Autodesk Inventor part; units mm, degrees
ref_plane "YZ Plane" through (0, 0, 0) normal (1, 0, 0) x (0, 1, 0)
ref_plane "XZ Plane" through (0, 0, 0) normal (0, 1, 0) x (-1, 0, 0)
ref_plane "XY Plane" through (0, 0, 0) normal (0, 0, 1) x (1, 0, 0)
sketch "Sketch1" plane through (0, 0, 0) normal (0, 0, 1) x (1, 0, 0)
  line L0 (-127, 635) -> (127, 635)
  line L1 (127, 635) -> (127, -635)
  line L2 (127, -635) -> (-127, -635)
  line L3 (-127, -635) -> (-127, 635)
  line L4 (-127, 635) -> (127, -635) construction
  line L5 (127, 635) -> (-127, -635) construction
  point P0 (0, 0)
  dimension "d0" = 254
  dimension "d1" = 1270
extrude "Extrusion1" add sketch "Sketch1" along normal blind 25.4
sketch "Sketch2" plane through (0, 0, 25.4) normal (0, 0, 1) x (1, 0, 0)
  line L0 (127, 635) -> (-127, 635)
  line L1 (-63.5, -381) -> (63.5, -381)
  line L2 (63.5, -381) -> (63.5, -508)
  line L3 (63.5, -508) -> (-63.5, -508)
  line L4 (-63.5, -508) -> (-63.5, -381)
  line L5 (-63.5, -381) -> (63.5, -508) construction
  line L6 (63.5, -381) -> (-63.5, -508) construction
  line L7 (0, 635) -> (0, 508)
  point P0 (0, 0)
  dimension "d5" = 127
  dimension "d6" = 127
  dimension "d7" = 127
hole "Hole1" at (0, 508, 25.4) direction (0, 0, -1) diameter 6.35 end through all
extrude "Extrusion2" add sketch "Sketch2" along normal blind 254
sketch "Sketch3" plane through (-63.5, -381, 25.4) normal (0, 1, 0) x (1, 0, 0)
  line L0 (127, -254) -> (0, -254)
  line L1 (127, 0) -> (127, -254)
  line L2 (63.5, -254) -> (63.5, -50.8)
  point P0 (63.5, 25.4)
  dimension "d17" = 203.2
hole "Hole2" at (0, -381, 76.2) direction (0, -1, 0) diameter 6.35 end through all
sketch "Sketch4" plane through (-63.5, -381, 25.4) normal (0, 1, 0) x (1, 0, 0)
  circle A0 centre (63.5, -50.8) radius 3.175
  line L0 (0, 0) -> (127, 0)
  line L1 (0, 0) -> (0, -254)
  line L2 (127, -254) -> (0, -254)
  line L3 (127, 0) -> (127, -254)
  point P0 (63.5, 25.4)
  point P1 (63.5, -53.975)
properties part number "base"
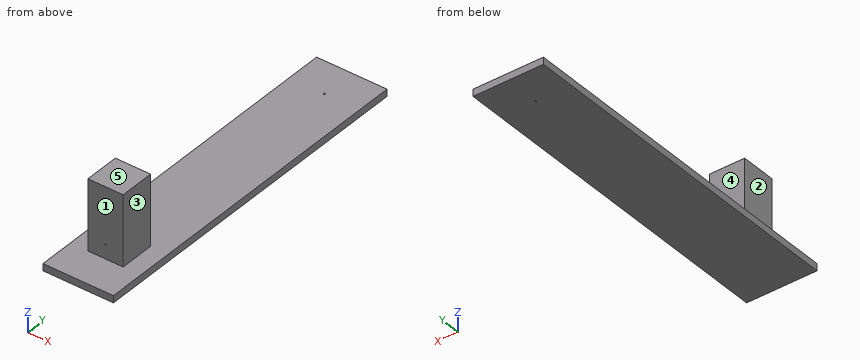
Input: part model. Units: mm. Frame: model coordinates. Face numbers are marked on the shaded views. A direction names the side the tool comes from. Coordinates: 2 decimals unless noted, no trailing zeros. Order: outer loops, then holes, each group sorted by start corner. A loop starts at its lowest first (then second) coordinate and runs counter-clockwise, first axis right, second up. Notation, with made-up numbers: M 36.5,81 L 58.5,81 A10 ccw 58.5,94 Z; hole C -29.75,15 d4. An arc over 180 degrees is marked long. Write item = value, one per line. Start each with the question number.
(1) Section D-D on y = -347.5. Output: boundary loops of the cut face in (x, z).
(2) Section A-A on y = -491.5. Output: boundary loops of the cut face in (x, z) (3 decimals), and give its area (3 significant figures).
(3) Line query: line 1 along Y through (x, z) = (0, 20) (3 decimals); line 2 along X through (y, z) = (508, 8.75) (3 decimals); line 3 along Z through (x, y) = (42, 519.5). Output: solid intervals per line, ascending. Write a range as [from, to].
(4) First-contact query: P1, Ø3, axis at x = 0.5, y = -244, coming from the +Z side. Flat tip, straight axial feed; report the tip coordinate or a pass-through.
(5) Section C-C on z = 216.5. Output: boundary loops of the cut face in (x, y).
(6) Reachability of the marked faces 1, 2, 3, 4 and 5 from +Z, -Z, +X, -X, +Y, -Y: full face, straight path, thin tool, end or side. Return the list, or none.
(7) Section B-B on x = -31. Output: boundary loops of the cut face in (y, z), and give its area (3 significant figures).
Result set:
q1.outline = M -127,0 L 127,0 L 127,25.4 L -127,25.4 Z
q2.outline = M -127,0 L 127,0 L 127,25.4 L 63.5,25.4 L 63.5,279.4 L -63.5,279.4 L -63.5,25.4 L -127,25.4 Z; hole C 0,76.2 d6.35
q2.area = 38,700 mm²
q3.line_1 = [-635, 504.825], [511.175, 635]
q3.line_2 = [-127, -3.175], [3.175, 127]
q3.line_3 = [0, 25.4]
q4.P1 = 25.4
q5.outline = M -63.5,-508 L 63.5,-508 L 63.5,-381 L -63.5,-381 Z
q6.face_1 = +Z, +X, -X, -Y
q6.face_2 = +Z, -X, +Y, -Y
q6.face_3 = +Z, +X, +Y, -Y
q6.face_4 = +Z, +X, -X, +Y
q6.face_5 = +Z, +X, -X, +Y, -Y
q7.outline = M -635,0 L 635,0 L 635,25.4 L -381,25.4 L -381,279.4 L -508,279.4 L -508,25.4 L -635,25.4 Z
q7.area = 64,500 mm²
